from build123d import *

# Parameters (mm, degrees)
F0_W     = 150
F0_H     = 80
F1_DEPTH = 12
F2_W     = 142
F2_H     = 8
F3_DEPTH = 3
F4_W     = 107.76
F4_H     = 12.85
F4_H_2   = 53.15
F4_W_2   = 28.24
F5_DEPTH = 7
F6_R     = 2


with BuildPart() as f1:
    # F0 (on Top) → F1 (new body)
    with BuildSketch(Plane.XY):
        with Locations((75, 40)):
            Rectangle(F0_W, F0_H)
    extrude(amount=F1_DEPTH)

    # F2 (on face) → F3 (join)
    with BuildSketch(Plane.XY.offset(12)):
        Polygon((0, 80), (0, 0), (8, 0), (8, 8), (8, 80), align=None)
        with Locations((79, 4)):
            Rectangle(F2_W, F2_H)
    extrude(amount=F3_DEPTH)

    # F4 (on face) → F5 (cut)
    with BuildSketch(Plane.XY.offset(12)):
        with Locations((63.88, 73.575)):
            Rectangle(F4_W, F4_H)
        with Locations((63.88, 36.575)):
            Rectangle(F4_W, F4_H_2)
        with Locations((135.88, 36.575)):
            Rectangle(F4_W_2, F4_H_2)
        with Locations((135.88, 73.575)):
            Rectangle(F4_W_2, F4_H)
    extrude(amount=-F5_DEPTH, mode=Mode.SUBTRACT)

    # F6
    f6_edges = [f1.edges().sort_by_distance(p)[0] for p in [
        (10, 63.15, 8.5),
        (117.76, 63.15, 8.5),
        (121.76, 63.15, 8.5),
        (121.76, 67.15, 8.5),
        (117.76, 67.15, 8.5),
        (117.76, 10, 8.5),
        (10, 10, 8.5),
        (10, 67.15, 8.5),
        (121.76, 10, 8.5),
    ]]
    fillet(f6_edges, radius=F6_R)


solid = f1.part
Design review of the part built by this model. Coordinates are the model's own, in mm. A direction names the side the tool comes from. Give positions to 0.01 mm unless a question says otherwise; leave off trailing zeros. Order: outer loops, then holes, each group sorted by start corner. A loop starts at its lowest first (then second) coordinate and runs counter-clockwise, first axis right, second up.
1. Add section B-B, the plane y = 15. State the section outline as (x, z) points.
Solution:
outline: (0, 0) - (150, 0) - (150, 5) - (121.76, 5) - (121.76, 12) - (117.76, 12) - (117.76, 5) - (10, 5) - (10, 12) - (8, 12) - (8, 15) - (0, 15) - close
2. Mouldability with a two-part tool opening along Y and no side actions: class faces 4 (the flat face through (0, 41, 7)), 5 (the flat face through (63, 63.15, 9)), 6 (the flat face through (74, 0, 7)) as +Y half, -Y half, draft (parallel to the pull), parting line (faces both ways), or undercut.
Solution:
face 4: draft
face 5: undercut
face 6: -Y half
3. Add section A-A, the plane z = 9. State the section outline as (x, y) points.
Solution:
outline: (0, 0) - (150, 0) - (150, 10) - (123.76, 10) arc R2 cw to (121.76, 12) - (121.76, 61.15) arc R2 cw to (123.76, 63.15) - (150, 63.15) - (150, 67.15) - (123.76, 67.15) arc R2 cw to (121.76, 69.15) - (121.76, 80) - (117.76, 80) - (117.76, 69.15) arc R2 cw to (115.76, 67.15) - (12, 67.15) arc R2 cw to (10, 69.15) - (10, 80) - (0, 80) - close; hole (10, 12) arc R2 ccw to (12, 10) - (115.76, 10) arc R2 ccw to (117.76, 12) - (117.76, 61.15) arc R2 ccw to (115.76, 63.15) - (12, 63.15) arc R2 ccw to (10, 61.15) - close
4. To check wall thickness, follow L1, parallel to Y at x = 74, z = 10.75; L2, parallel to X at y = 15, z = 5.75; L3, parallel to Y at x = 45.5, z = 13.5. State the ranges of each line that lie inside material, in increasing order.
Solution:
L1: y = 0 to 10, 63.15 to 67.15
L2: x = 0 to 10, 117.76 to 121.76
L3: y = 0 to 8
5. Tool access review of faces 1 (the flat face through (117.76, 74, 9)), 2 (the flat face through (121.76, 36, 9)), 3 (the flat face through (89, 66, 12)): name each direction out of +Z, -Z, +X, -X, +Y, -Y from which nothing blocks a thin tool from reaching the whole face with its end or side.
Solution:
face 1: +Z, +Y
face 2: +Z, +X
face 3: +Z, +X, +Y
6. For pin 1 Ø7.5 at (x, z) = (78.5, 8) entering from -Y; pin 2 Ø2.5 at (x, z) = (87.5, 13.5) entering from +Y; pin 3 Ø2 at (y, z) = (48, 7.5) entering from +X; pin 4 Ø2 at (x, z) = (58.5, 8.5) entering from +Y, all flat-tipped, find the tip position at first contact; note any pin that passes through.
Solution:
pin 1: stops at y = 0
pin 2: stops at y = 8
pin 3: stops at x = 121.76
pin 4: stops at y = 67.15
7. Add section C-C, the plane x = 22. State the section outline as (y, z) points.
Solution:
outline: (0, 0) - (80, 0) - (80, 5) - (67.15, 5) - (67.15, 12) - (63.15, 12) - (63.15, 5) - (10, 5) - (10, 12) - (8, 12) - (8, 15) - (0, 15) - close
